Autodesk Inventor part; units mm, degrees
ref_plane "YZ Plane" through (0, 0, 0) normal (1, 0, 0) x (0, 1, 0)
ref_plane "XZ Plane" through (0, 0, 0) normal (0, 1, 0) x (-1, 0, 0)
ref_plane "XY Plane" through (0, 0, 0) normal (0, 0, 1) x (1, 0, 0)
sketch "Sketch2" plane through (0, 0, 0) normal (0, 0, 1) x (1, 0, 0)
  line L0 (0, 0) -> (-9.9, 0)
  line L1 (-9.9, 0) -> (-9.9, 105)
  line L2 (-9.9, 105) -> (0, 105)
  line L3 (0, 105) -> (0, 0)
  line L4 (-4.95, 0) -> (-4.95, 2.5)
  line L5 (-4.95, 0) -> (-2.45, 0) construction
  circle A0 centre (-4.95, 5) radius 2.5
  line L6 (-4.95, 7.5) -> (32.05, 7.5) construction
  line L7 (0, 44.5) -> (0, 0)
  line L8 (0, 0) -> (-9.9, 0)
  line L9 (-9.9, 0) -> (-9.9, 44.5)
  line L10 (-9.9, 45.5) -> (0, 45.5)
  line L11 (0, 45.5) -> (0, 0)
  line L12 (0, 0) -> (-9.9, 0)
  line L13 (-9.9, 0) -> (-9.9, 45.5)
  dimension "d35" = 5
  dimension "d4" = 9.9
  dimension "d5" = 105
  dimension "d33" = 2.5
  dimension "d34" = 90
extrude "Extrusion5" add sketch "Sketch2" along normal blind 5 contours L0 L1 L10 L3
properties part number "Cube_Holder_EB_V2_(38mm)"
Model file for the job. Use its own axes, mm. Give positions to 0.01 mm unless a question says otherwise; leave off trailing zeros. Order: outer loops, then holes, each group sorted by start corner. A loop starts at its lowest first (then second) coordinate and runs counter-clockwise, first axis right, second up. Notation, with made-up numbers: M 36.5,85 L 79.5,85 A23 cw 79.5,123 Z; hole C 74.5,-24 d7. An arc over 180 degrees is marked long. Put each result on its own line as item: value. Start each with the question number.
(1) Pull direction Y, two halves, no side cores. Call faces 1 (the face through (-5, 0, 2)), 2 (the face through (0, 23, 2)), 3 (the face through (-2.565, 4.249, 2.465)), 4 (the face through (-5, 45.5, 2)): released by +Y, released by -Y, zero draft, split by the parting line, or undercut.
(2) Band-saw the part on A-A on y = 5. Give the cut face in (x, z), then the cut area to 3 significant figures.
(3) Drill centre lines: L1, parallel to Y at x = -4.95, z = 3.65; L2, parallel to X at y = 5, z = 2.45; L3, parallel to X at y = 6, z = 2.7. Where is each one in solid material? Low to high. Write a range as [from, to].
(4) Band-saw the part on C-C on z = 3. Give the cut face in (x, y).
(5) Band-saw the part on B-B on x = -4.95. Give the cut face in (y, z), then the cut area to 4 significant figures.
Results below:
1. face 1: released by -Y
1. face 2: zero draft
1. face 3: undercut
1. face 4: released by +Y
2. outline: M -9.9,0 L -7.45,0 L -7.45,5 L -9.9,5 Z; M -2.45,0 L 0,0 L 0,5 L -2.45,5 Z
2. area: 24.5 mm2
3. L1: y = [0, 2.5], [7.5, 45.5]
3. L2: x = [-9.9, -7.45], [-2.45, 0]
3. L3: x = [-9.9, -7.24], [-2.66, 0]
4. outline: M -9.9,0 L 0,0 L 0,45.5 L -9.9,45.5 Z; hole C -4.95,5 d5
5. outline: M 0,0 L 2.5,0 L 2.5,5 L 0,5 Z; M 7.5,0 L 45.5,0 L 45.5,5 L 7.5,5 Z
5. area: 202.5 mm2
